The figure shows three views and two pictorial views of one solid part (mm, origin at its lowest corner). Answer the questions. Round coordinates to 2 decimals unless told otherwise and drop trailing zeros. Write each loop counter-clockwise with the first axis right and the second up, starting at its lowest first coordinate (ties: lowest second). Pieces come first, ordered by that corner, then holes. Notation, with made-up numbers: (-36, 87.25) - (-20, 87.25) arc R22 ccw to (-20, 125.25) - close; hole circle Ø10 at (24.25, 60). An arc over 180 degrees is marked (long way). Answer as CSV lines item,"result". Start each with the question number.
Item 1: A cutting plane is placed at A-A on y = 16. Determine the outline of the cut face in (x, z), and give its area (3 significant figures).
Item 2: Straight lines are drawn through the part: line 1 along Y through (x, z) = (11.25, 2.25); line 2 along Z through (x, y) = (14.25, 15). For each, find the intervals that lie inside material, in ascending order. Write a range as [from, to].
Item 3: Flat-ended cylindrical pins translate along their axes: pin 1 (1.8 mm diameter, centred on x = 9.25, y = 9.25, fed in from -Z); pin 2 (1 mm diameter, centred on y = 10.5, z = 1, fed in from +X); pin 3 (1 mm diameter, centred on y = 11, z = 1, fed in from -X); pin 4 (2 mm diameter, centred on y = 13.5, z = 1, fed in from -X). Find the tip coordinate at first contact, or state that the pin passes through.
Item 4: For a pull along X with two mould halves and no side action, classify the marked faces 1, 2, 3 and 4 as pulls with the +X half, pulls with the -X half, needs draft (parallel to the pull), parting line crosses it, or undercut.
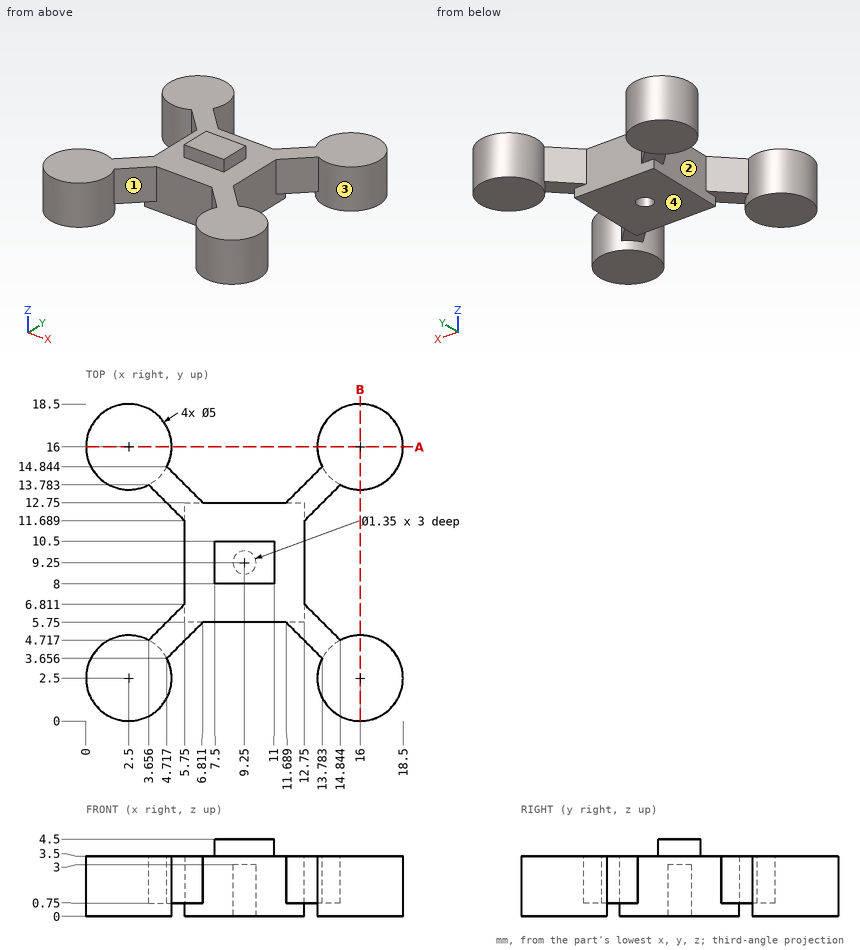
Geometry says:
1,outline,"(0, 0) - (5, 0) - (5, 3.5) - (0, 3.5) - close; (13.5, 0) - (18.5, 0) - (18.5, 3.5) - (13.5, 3.5) - close"
1,area,"35.0 mm^2"
2,line 1,"y = [5.75, 12.75]"
2,line 2,"z = [0, 3.5]"
3,pin 1,"stops at z = 0"
3,pin 2,"stops at x = 12.75"
3,pin 3,"stops at x = 5.75"
3,pin 4,"stops at x = 0.5"
4,face 1,"undercut"
4,face 2,"pulls with the -X half"
4,face 3,"undercut"
4,face 4,"needs draft"
